Check sheet for the drawn part. Datum: minimum x, y, z corner. Units: mm. A direction names the side the tool comes from. Round coordinates to 2 decimals unless told otherwise and drop trailing zeros. Write each loop counter-clockwise with the first axis right and the second up, starting at its lowest first coordinate (ties: lowest second). Pieces come first, ordered by that corner, then holes. Notation, with made-up numbers: (-12, 36) - (11, 36) arc R12 ccw to (11, 47) - close; hole circle Ø1 at (-34, 53.5). An arc over 180 degrees is marked (long way). Answer as a JSON object with one key per item and string values. Group by question number.
1) Thickness scan on line 1 (Z direction, x = 22.5, y = 8); line 2 (X direction, y = 5, z = 5.5); line 3 (Z direction, x = 20.5, y = 4). Record the ranges inside material, lowest first.
2) Mould release check, pull along X, two halves, no side actions. Record for the marked faces 1, 2 and 3: +X half, -X half, draft (parallel to the pull), parting line (faces both ways), or undercut.
3) Go/stop test with flat-tipped pins: pin 1 Ø1.5 at (x, y) = (6, 4.5) entering from -Z; pin 2 Ø7 at (x, z) = (20, 37) entering from +Y. Record where each tip stops, or that it passes through.
4) Section check A-A (x = 22.5). Enter the section's corners in (y, z), then the cut area to 3 significant figures.
5) Set-up check for the marked faces 4 and 5: record each of +Z, -Z, +X, -X, +Y, -Y from which the full face is reachable in a straight line by a thin tool's end or side.
6) Section check C-C (y = 5.75). Enter the section's corners in (x, z), then the cut area to 3 significant figures.
7) Section check B-B (y = 1.25). Enter the section's corners in (x, z), then the cut area to 3 significant figures.
8) Section check D-D (z = 9). Enter the section's corners in (x, y), then the cut area to 3 significant figures.
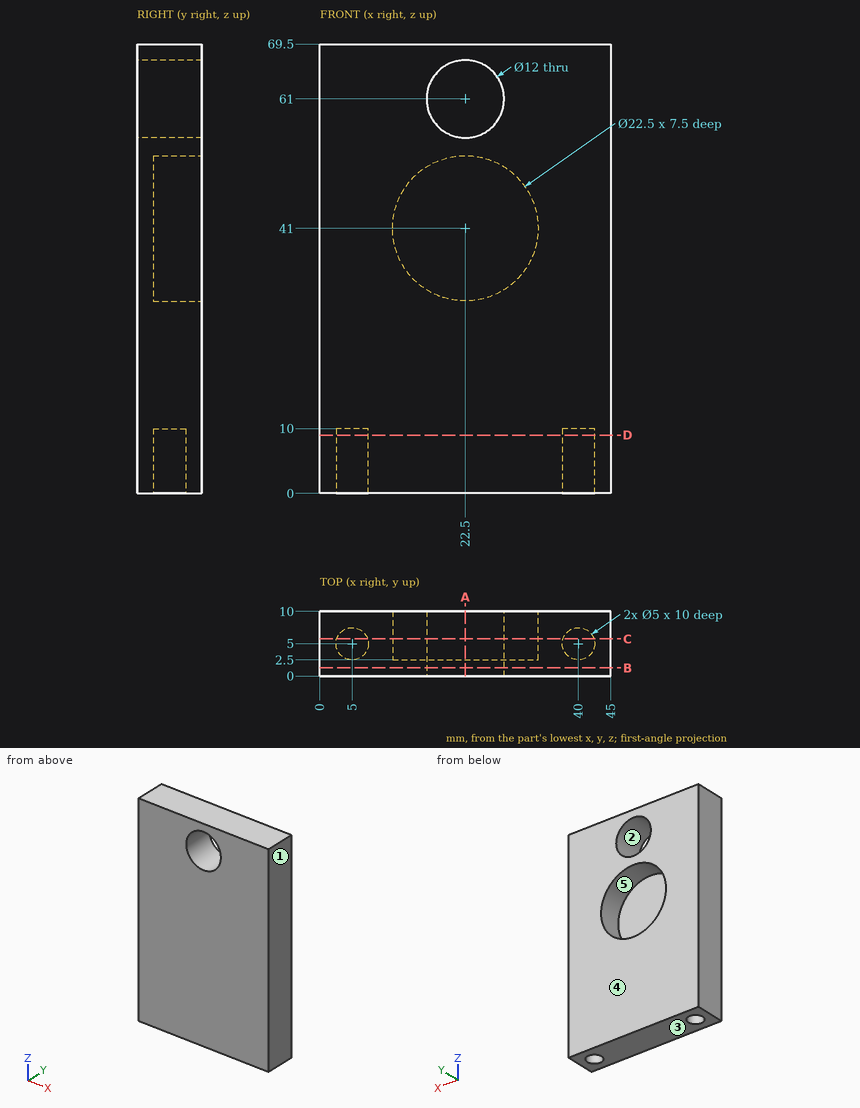
Returned:
{
 "1": {"line 1": "0 to 29.75, 52.25 to 55, 67 to 69.5", "line 2": "0 to 2.5, 7.5 to 37.5, 42.5 to 45", "line 3": "0 to 29.93, 52.07 to 55.34, 66.66 to 69.5"},
 "2": {"face 1": "+X half", "face 2": "undercut", "face 3": "draft"},
 "3": {"pin 1": "z = 10", "pin 2": "y = 2.5"},
 "4": {"outline": "(0, 0) - (10, 0) - (10, 29.75) - (2.5, 29.75) - (2.5, 52.25) - (10, 52.25) - (10, 55) - (0, 55) - close; (0, 67) - (10, 67) - (10, 69.5) - (0, 69.5) - close", "area": "406 mm2"},
 "5": {"face 4": "+Z, -Z, +X, -X, +Y", "face 5": "+Y"},
 "6": {"outline": "(0, 0) - (2.62, 0) - (2.62, 10) - (7.38, 10) - (7.38, 0) - (37.62, 0) - (37.62, 10) - (42.38, 10) - (42.38, 0) - (45, 0) - (45, 69.5) - (0, 69.5) - close; hole circle Ø22.5 at (22.5, 41); hole circle Ø12 at (22.5, 61)", "area": "2,520 mm2"},
 "7": {"outline": "(0, 0) - (45, 0) - (45, 69.5) - (0, 69.5) - close; hole circle Ø12 at (22.5, 61)", "area": "3,010 mm2"},
 "8": {"outline": "(0, 0) - (45, 0) - (45, 10) - (0, 10) - close; hole circle Ø5 at (5, 5); hole circle Ø5 at (40, 5)", "area": "411 mm2"}
}
